```python
from build123d import *

# Parameters (mm, degrees)
SKICA1_W                 = 16
SKICA1_H                 = 16
P_IDAT_VYSUNUT_M1_DEPTH  = 7
SKICA2_W                 = 17.85
SKICA2_H                 = 54.1
P_IDAT_VYSUNUT_M2_DEPTH  = 4
SKICA3_W                 = 7.868538626
SKICA3_H                 = 3.04290642
SKICA3_W_2               = 8
SKICA3_H_2               = 2.219116854
SKICA3_H_3               = 2.772139553
SKICA3_H_4               = 2.562795671
ODEBRAT_VYSUNUT_M1_DEPTH = 3
ZAOBLIT1_R               = 0.5
ZAOBLIT2_R               = 1.7


with BuildPart() as part:
    # Skica1 → Přidat vysunutím1 (new body)
    with BuildSketch(Plane.XY):
        with BuildLine():
            Line((-7.5, 47.3), (64.65, 47.3))
            ThreePointArc((64.65, 47.3), (65.852081528, 46.802081528), (66.35, 45.6))
            Line((66.35, 45.6), (66.35, -7.5))
            ThreePointArc((66.35, -7.5), (65.852081528, -8.702081528), (64.65, -9.2))
            Line((64.65, -9.2), (-7.5, -9.2))
            ThreePointArc((-7.5, -9.2), (-8.702081528, -8.702081528), (-9.2, -7.5))
            Line((-9.2, -7.5), (-9.2, 45.6))
            ThreePointArc((-9.2, 45.6), (-8.702081528, 46.802081528), (-7.5, 47.3))
        make_face()
        with Locations((19.05, 0)):
            Rectangle(SKICA1_W, SKICA1_H, mode=Mode.SUBTRACT)
        with BuildLine():
            Line((-8, 8), (8, 8))
            Line((8, 8), (8, -8))
            Line((8, -8), (-7.5, -8))
            ThreePointArc((-7.5, -8), (-7.853553391, -7.853553391), (-8, -7.5))
            Line((-8, -7.5), (-8, 8))
        make_face(mode=Mode.SUBTRACT)
        with Locations((38.1, 0)):
            Rectangle(SKICA1_W, SKICA1_H, mode=Mode.SUBTRACT)
        with BuildLine():
            Line((49.15, 8), (49.15, -8))
            Line((49.15, -8), (64.65, -8))
            ThreePointArc((64.65, -8), (65.003553391, -7.853553391), (65.15, -7.5))
            Line((65.15, -7.5), (65.15, 8))
            Line((65.15, 8), (49.15, 8))
        make_face(mode=Mode.SUBTRACT)
        with Locations((19.05, 19.05)):
            Rectangle(SKICA1_W, SKICA1_H, mode=Mode.SUBTRACT)
        with Locations((38.1, 19.05)):
            Rectangle(SKICA1_W, SKICA1_H, mode=Mode.SUBTRACT)
        with Locations((57.15, 19.05)):
            Rectangle(SKICA1_W, SKICA1_H, mode=Mode.SUBTRACT)
        with Locations((19.05, 38.1)):
            Rectangle(SKICA1_W, SKICA1_H, mode=Mode.SUBTRACT)
        with Locations((38.1, 38.1)):
            Rectangle(SKICA1_W, SKICA1_H, mode=Mode.SUBTRACT)
        with BuildLine():
            Line((49.15, 46.1), (49.15, 30.1))
            Line((49.15, 30.1), (65.15, 30.1))
            Line((65.15, 30.1), (65.15, 45.6))
            ThreePointArc((65.15, 45.6), (65.003553391, 45.953553391), (64.65, 46.1))
            Line((64.65, 46.1), (49.15, 46.1))
        make_face(mode=Mode.SUBTRACT)
        with Locations((0, 19.05)):
            Rectangle(SKICA1_W, SKICA1_H, mode=Mode.SUBTRACT)
        with BuildLine():
            Line((-8, 45.6), (-8, 30.1))
            Line((-8, 30.1), (8, 30.1))
            Line((8, 30.1), (8, 46.1))
            Line((8, 46.1), (-7.5, 46.1))
            ThreePointArc((-7.5, 46.1), (-7.853553391, 45.953553391), (-8, 45.6))
        make_face(mode=Mode.SUBTRACT)
    extrude(amount=P_IDAT_VYSUNUT_M1_DEPTH)

    # Skica2 → Přidat vysunutím2 (add)
    with BuildSketch(Plane.XY.offset(7)):
        with BuildLine():
            Line((-7.5, -9.2), (64.65, -9.2))
            ThreePointArc((64.65, -9.2), (65.852081528, -8.702081528), (66.35, -7.5))
            Line((66.35, -7.5), (66.35, 45.6))
            ThreePointArc((66.35, 45.6), (65.852081528, 46.802081528), (64.65, 47.3))
            Line((64.65, 47.3), (-7.5, 47.3))
            ThreePointArc((-7.5, 47.3), (-8.702081528, 46.802081528), (-9.2, 45.6))
            Line((-9.2, 45.6), (-9.2, -7.5))
            ThreePointArc((-9.2, -7.5), (-8.702081528, -8.702081528), (-7.5, -9.2))
        make_face()
        with BuildLine():
            Line((64.65, 46.1), (48.125, 46.1))
            Line((48.125, 46.1), (48.125, -8))
            Line((48.125, -8), (64.65, -8))
            ThreePointArc((64.65, -8), (65.003553391, -7.853553391), (65.15, -7.5))
            Line((65.15, -7.5), (65.15, 45.6))
            ThreePointArc((65.15, 45.6), (65.003553391, 45.953553391), (64.65, 46.1))
        make_face(mode=Mode.SUBTRACT)
        with BuildLine():
            Line((-8, 45.6), (-8, -7.5))
            ThreePointArc((-8, -7.5), (-7.853553391, -7.853553391), (-7.5, -8))
            Line((-7.5, -8), (8.825, -8))
            Line((8.825, -8), (8.825, 46.1))
            Line((8.825, 46.1), (-7.5, 46.1))
            ThreePointArc((-7.5, 46.1), (-7.853553391, 45.953553391), (-8, 45.6))
        make_face(mode=Mode.SUBTRACT)
        with Locations((18.95, 19.05)):
            Rectangle(SKICA2_W, SKICA2_H, mode=Mode.SUBTRACT)
        with Locations((38, 19.05)):
            Rectangle(SKICA2_W, SKICA2_H, mode=Mode.SUBTRACT)
    extrude(amount=P_IDAT_VYSUNUT_M2_DEPTH)

    # Skica3 → Odebrat vysunutím1 (cut)
    with BuildSketch(Plane.XY.offset(11)):
        with Locations((-5.934269313, 47.141342461)):
            Rectangle(SKICA3_W, SKICA3_H)
        with Locations((14.025, 47.209558427)):
            Rectangle(SKICA3_W_2, SKICA3_H_2)
        with Locations((33.075, 47.486069777)):
            Rectangle(SKICA3_W_2, SKICA3_H_3)
        with Locations((52.125, 47.381397836)):
            Rectangle(SKICA3_W_2, SKICA3_H_4)
    extrude(amount=-ODEBRAT_VYSUNUT_M1_DEPTH, mode=Mode.SUBTRACT)

    # Zaoblit1
    zaoblit1_edges = [part.edges().sort_by_distance(p)[0] for p in [
        (8.825, 46.1, 9),
        (27.875, 46.1, 9),
        (46.925, 46.1, 9),
    ]]
    fillet(zaoblit1_edges, radius=ZAOBLIT1_R)

    # Zaoblit2
    # the kernel refuses this fillet: 1.7 mm, written as the material it takes off along each edge
    with BuildSketch(Plane(origin=(48.125, 47.3, 3.75), x_dir=(-1, 0, 0), z_dir=(0, 0, 1))) as zaoblit2_piece_1_section:
        with BuildLine():
            CenterArc((ZAOBLIT2_R, ZAOBLIT2_R), ZAOBLIT2_R, 180, 90)
            Line((0, ZAOBLIT2_R), (0, 0))
            Line((0, 0), (ZAOBLIT2_R, 0))
        make_face()
    zaoblit2_piece_1 = extrude(amount=11.5, mode=Mode.PRIVATE)
    zaoblit2_piece_1 = split(zaoblit2_piece_1, bisect_by=Plane(origin=(48.125338214, 45.903004102, 8), z_dir=(0, 0, -1)), keep=Keep.TOP, mode=Mode.PRIVATE)
    zaoblit2_piece_1 = split(zaoblit2_piece_1, bisect_by=Plane(origin=(48.125338214, 46.1, 7.5), z_dir=(0, -1, 0)), keep=Keep.TOP, mode=Mode.PRIVATE)
    zaoblit2_piece_1 = split(zaoblit2_piece_1, bisect_by=Plane(origin=(48.125338214, 45.903004102, 7), z_dir=(0, 0, 1)), keep=Keep.TOP, mode=Mode.PRIVATE)
    add(zaoblit2_piece_1, mode=Mode.SUBTRACT)
    with BuildSketch(Plane(origin=(48.125, 47.3, 8), x_dir=(-1, 0, 0), z_dir=(0, 0, 1))) as zaoblit2_piece_2_section:
        with BuildLine():
            CenterArc((ZAOBLIT2_R, ZAOBLIT2_R), ZAOBLIT2_R, 180, 90)
            Line((0, ZAOBLIT2_R), (0, 0))
            Line((0, 0), (ZAOBLIT2_R, 0))
        make_face()
    zaoblit2_piece_2 = extrude(amount=7.25, mode=Mode.PRIVATE)
    zaoblit2_piece_2 = split(zaoblit2_piece_2, bisect_by=Plane(origin=(47.724111446, 46.1, 11.625), z_dir=(0, 1, 0)), keep=Keep.TOP, mode=Mode.PRIVATE)
    add(zaoblit2_piece_2, mode=Mode.SUBTRACT)
    with BuildSketch(Plane(origin=(48.125, 47.3, 8), x_dir=(-1, 0, 0), z_dir=(0, 0, 1))) as zaoblit2_piece_3_section:
        with BuildLine():
            CenterArc((ZAOBLIT2_R, ZAOBLIT2_R), ZAOBLIT2_R, 180, 90)
            Line((0, ZAOBLIT2_R), (0, 0))
            Line((0, 0), (ZAOBLIT2_R, 0))
        make_face()
    zaoblit2_piece_3 = extrude(amount=7.25, mode=Mode.PRIVATE)
    zaoblit2_piece_3 = split(zaoblit2_piece_3, bisect_by=Plane(origin=(48.125338214, 46.1, 11.625), z_dir=(0, -1, 0)), keep=Keep.TOP, mode=Mode.PRIVATE)
    add(zaoblit2_piece_3, mode=Mode.SUBTRACT)
    with BuildSketch(Plane(origin=(29.075, 47.3, 3.75), x_dir=(-1, 0, 0), z_dir=(0, 0, 1))) as zaoblit2_piece_4_section:
        with BuildLine():
            CenterArc((ZAOBLIT2_R, ZAOBLIT2_R), ZAOBLIT2_R, 180, 90)
            Line((0, ZAOBLIT2_R), (0, 0))
            Line((0, 0), (ZAOBLIT2_R, 0))
        make_face()
    zaoblit2_piece_4 = extrude(amount=11.5, mode=Mode.PRIVATE)
    zaoblit2_piece_4 = split(zaoblit2_piece_4, bisect_by=Plane(origin=(29.075338214, 46.1, 7.5), z_dir=(0, -1, 0)), keep=Keep.TOP, mode=Mode.PRIVATE)
    zaoblit2_piece_4 = split(zaoblit2_piece_4, bisect_by=Plane(origin=(29.075338214, 45.903004102, 8), z_dir=(0, 0, -1)), keep=Keep.TOP, mode=Mode.PRIVATE)
    zaoblit2_piece_4 = split(zaoblit2_piece_4, bisect_by=Plane(origin=(29.075338214, 45.903004102, 7), z_dir=(0, 0, 1)), keep=Keep.TOP, mode=Mode.PRIVATE)
    add(zaoblit2_piece_4, mode=Mode.SUBTRACT)
    with BuildSketch(Plane(origin=(29.075, 47.3, 8), x_dir=(-1, 0, 0), z_dir=(0, 0, 1))) as zaoblit2_piece_5_section:
        with BuildLine():
            CenterArc((ZAOBLIT2_R, ZAOBLIT2_R), ZAOBLIT2_R, 180, 90)
            Line((0, ZAOBLIT2_R), (0, 0))
            Line((0, 0), (ZAOBLIT2_R, 0))
        make_face()
    zaoblit2_piece_5 = extrude(amount=7.25, mode=Mode.PRIVATE)
    zaoblit2_piece_5 = split(zaoblit2_piece_5, bisect_by=Plane(origin=(28.674111446, 46.1, 11.625), z_dir=(0, 1, 0)), keep=Keep.TOP, mode=Mode.PRIVATE)
    add(zaoblit2_piece_5, mode=Mode.SUBTRACT)
    with BuildSketch(Plane(origin=(29.075, 47.3, 8), x_dir=(-1, 0, 0), z_dir=(0, 0, 1))) as zaoblit2_piece_6_section:
        with BuildLine():
            CenterArc((ZAOBLIT2_R, ZAOBLIT2_R), ZAOBLIT2_R, 180, 90)
            Line((0, ZAOBLIT2_R), (0, 0))
            Line((0, 0), (ZAOBLIT2_R, 0))
        make_face()
    zaoblit2_piece_6 = extrude(amount=7.25, mode=Mode.PRIVATE)
    zaoblit2_piece_6 = split(zaoblit2_piece_6, bisect_by=Plane(origin=(29.075338214, 46.1, 11.625), z_dir=(0, -1, 0)), keep=Keep.TOP, mode=Mode.PRIVATE)
    add(zaoblit2_piece_6, mode=Mode.SUBTRACT)
    with BuildSketch(Plane(origin=(10.025, 47.3, 3.75), x_dir=(-1, 0, 0), z_dir=(0, 0, 1))) as zaoblit2_piece_7_section:
        with BuildLine():
            CenterArc((ZAOBLIT2_R, ZAOBLIT2_R), ZAOBLIT2_R, 180, 90)
            Line((0, ZAOBLIT2_R), (0, 0))
            Line((0, 0), (ZAOBLIT2_R, 0))
        make_face()
    zaoblit2_piece_7 = extrude(amount=11.5, mode=Mode.PRIVATE)
    zaoblit2_piece_7 = split(zaoblit2_piece_7, bisect_by=Plane(origin=(10.025338214, 46.1, 7.5), z_dir=(0, -1, 0)), keep=Keep.TOP, mode=Mode.PRIVATE)
    zaoblit2_piece_7 = split(zaoblit2_piece_7, bisect_by=Plane(origin=(10.025338214, 45.903004102, 8), z_dir=(0, 0, -1)), keep=Keep.TOP, mode=Mode.PRIVATE)
    zaoblit2_piece_7 = split(zaoblit2_piece_7, bisect_by=Plane(origin=(10.025338214, 45.903004102, 7), z_dir=(0, 0, 1)), keep=Keep.TOP, mode=Mode.PRIVATE)
    add(zaoblit2_piece_7, mode=Mode.SUBTRACT)
    with BuildSketch(Plane(origin=(10.025, 47.3, 8), x_dir=(-1, 0, 0), z_dir=(0, 0, 1))) as zaoblit2_piece_8_section:
        with BuildLine():
            CenterArc((ZAOBLIT2_R, ZAOBLIT2_R), ZAOBLIT2_R, 180, 90)
            Line((0, ZAOBLIT2_R), (0, 0))
            Line((0, 0), (ZAOBLIT2_R, 0))
        make_face()
    zaoblit2_piece_8 = extrude(amount=7.25, mode=Mode.PRIVATE)
    zaoblit2_piece_8 = split(zaoblit2_piece_8, bisect_by=Plane(origin=(9.624111446, 46.1, 11.625), z_dir=(0, 1, 0)), keep=Keep.TOP, mode=Mode.PRIVATE)
    add(zaoblit2_piece_8, mode=Mode.SUBTRACT)
    with BuildSketch(Plane(origin=(10.025, 47.3, 8), x_dir=(-1, 0, 0), z_dir=(0, 0, 1))) as zaoblit2_piece_9_section:
        with BuildLine():
            CenterArc((ZAOBLIT2_R, ZAOBLIT2_R), ZAOBLIT2_R, 180, 90)
            Line((0, ZAOBLIT2_R), (0, 0))
            Line((0, 0), (ZAOBLIT2_R, 0))
        make_face()
    zaoblit2_piece_9 = extrude(amount=7.25, mode=Mode.PRIVATE)
    zaoblit2_piece_9 = split(zaoblit2_piece_9, bisect_by=Plane(origin=(10.025338214, 46.1, 11.625), z_dir=(0, -1, 0)), keep=Keep.TOP, mode=Mode.PRIVATE)
    add(zaoblit2_piece_9, mode=Mode.SUBTRACT)


solid = part.part
```
CAD build for the part. Positions are in the model's coordinates, mm. A direction names the side the tool comes from. Round coordinates to 2 decimals unless told otherwise and drop trailing zeros. Order: outer loops, then holes, each group sorted by start corner. A loop starts at its lowest first (then second) coordinate and runs counter-clockwise, first axis right, second up. Notation, with made-up numbers: (-33, 33) - (-14, 33) arc R26 ccw to (-14, 68) - close; hole circle Ø7 at (26, 39.5). An arc over 180 degrees is marked (long way). Answer as CSV lines item,"result". Start each with the question number.
1. Saw through at A-A, the plane x = 40. Write the cut outline in (y, z), and give its area (3 significant figures).
2. Saw through at B-B, the plane y = 17. Count the separate pieces of the cut face and the enclosed holes in it, and give its area (3 significant figures).
3. Drill centre lines: L1, parallel to X at y = 44.5, z = 4; L2, parallel to Y at x = 6.5, z = 5.5; L3, parallel to X at y = 36.5, z = 10.5 (3 decimals). Where is each one in solid material? Low to high. Write a range as [from, to].
4. Pull direction X, two halves, no side cores. Call faces 4 (the face through (1, 46.1, 5)), 5 (the face through (-8.715, -8.689, 5.423)), 6 (the face through (-6, 47, 8)): +X half, -X half, draft (parallel to the pull), parting line (faces both ways), or undercut.
5. Pin check, flat tip, straight feed: pin 1 (13.5 mm diameter, centred on x = 2, y = 10.5, fed in from +Z). Stop position of the tip, or through.
6. Tool access for faces 1 (the face through (0, 8, 3)), 2 (the face through (48.4, 21.2, 7)), 3 (the face through (28.4, 15, 11)): list every direction of +Z, -Z, +X, -X, +Y, -Y with a clear straight run to the whole face (end or side of a thin tool).
7. Saw through at D-D, the plane x = 15.5. Write the cut outline in (y, z), and give its area (3 significant figures).
Model answer:
1,outline,"(-9.2, 0) - (-8, 0) - (-8, 11) - (-9.2, 11) - close; (8, 0) - (11.05, 0) - (11.05, 7) - (8, 7) - close; (27.05, 0) - (30.1, 0) - (30.1, 7) - (27.05, 7) - close; (46.1, 0) - (47.3, 0) - (47.3, 11) - (46.1, 11) - close"
1,area,"69.1 mm²"
2,separate pieces,"5"
2,enclosed holes,"0"
2,area,"105 mm²"
3,L1,"x = [-9.2, -8], [8, 11.05], [27.05, 30.1], [46.1, 49.15], [65.15, 66.35]"
3,L2,"y = [-9.2, -8], [8, 11.05], [27.05, 30.1], [46.1, 47.3]"
3,L3,"x = [-9.2, -8], [8.825, 10.025], [27.875, 29.075], [46.925, 48.125], [65.15, 66.35]"
4,face 4,"undercut"
4,face 5,"-X half"
4,face 6,"draft"
5,pin 1,"stops at z = 7"
6,face 1,"+Z, -Z"
6,face 2,"+Z"
6,face 3,"+Z, +X, -X, +Y, -Y"
7,outline,"(-9.2, 0) - (-8, 0) - (-8, 11) - (-9.2, 11) - close; (8, 0) - (11.05, 0) - (11.05, 7) - (8, 7) - close; (27.05, 0) - (30.1, 0) - (30.1, 7) - (27.05, 7) - close; (46.1, 0) - (47.3, 0) - (47.3, 8) - (46.1, 8) - close"
7,area,"65.5 mm²"
